Input: part model. Units: mm. Frame: model coordinates. Give positions to 0.01 mm unless a question says otherwise; leave off trailing zeros. Loops run counter-clockwise (first coordinate to the right, second up) from the corner with the lowest first, then second, coordinate; pieces in that order, holes last. Notation, with made-up numbers: (-6, 6.5) -> (5, 6.5) arc R15 cw to (5, 25.5) -> close; hole circle Ø2 at (-7, -15.5). An arc over 180 degrees is marked (long way). Answer as a JSON object with one key per item and string values. Group by question number.
```python
from build123d import *

# Parameters (mm, degrees)
SKETCH1_W           = 38.1
SKETCH1_H           = 406.4
BOSS_EXTRUDE1_DEPTH = 6.35
SKETCH2_W           = 6.35
SKETCH2_H           = 12.7
CUT_EXTRUDE1_DEPTH  = 7.35
LPATTERN1_COUNT     = 16
LPATTERN1_PITCH     = 25.4


with BuildPart() as part:
    # Sketch1 → Boss-Extrude1 (new body)
    with BuildSketch(Plane(origin=(0, 0, 0), x_dir=(0, 0, -1), z_dir=(1, 0, 0))):
        with Locations((19.05, 203.2)):
            Rectangle(SKETCH1_W, SKETCH1_H)
    extrude(amount=BOSS_EXTRUDE1_DEPTH)

    # Sketch2 → Cut-Extrude1 (cut, through all)
    with BuildSketch(Plane(origin=(6.35, 0, 0), x_dir=(0, 0, -1), z_dir=(1, 0, 0))):
        with Locations((3.175, 6.35)):
            Rectangle(SKETCH2_W, SKETCH2_H)
        with Locations((34.925, 6.35)):
            Rectangle(SKETCH2_W, SKETCH2_H)
    cut_extrude1 = extrude(amount=-CUT_EXTRUDE1_DEPTH, mode=Mode.SUBTRACT)

    # LPattern1: Cut-Extrude1 ×16
    with Locations(*[(0, i * LPATTERN1_PITCH, 0) for i in range(1, LPATTERN1_COUNT)]):
        add(cut_extrude1, mode=Mode.SUBTRACT)


solid = part.part
```
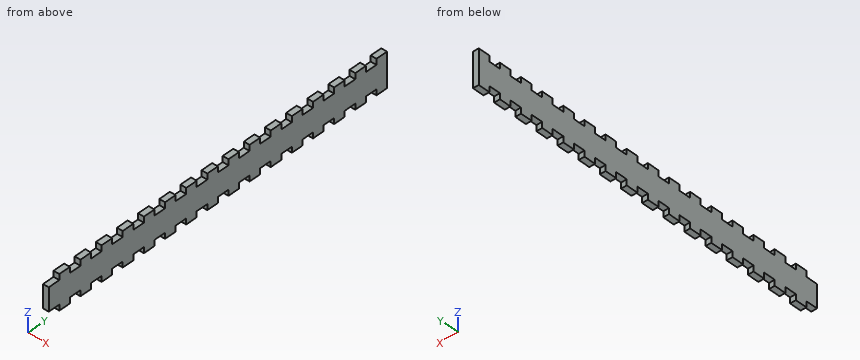
Q1. Pin query (flat end, axial travel): pin 1 Ø1 at (x, y) = (2, 207) entering from +Z; pin 2 Ø2 at (y, z) = (345.5, -17.5) entering from -X; pin 3 Ø3 at (x, z) = (4.5, -3) entering from -Y. Return the tip coordinate at first contact, or that it passes through.
Q2. Ray query, probe 1 along Z at (x, y) = (3.25, 154). Return the intervals inside material, ascending.
Q3. Section A-A on y = 261.5. Return the cut outline in (x, z), then the cut area to 3 significant figures.
Numbers:
{
 "1": {"pin 1": "stops at z = -6.35", "pin 2": "stops at x = 0", "pin 3": "stops at y = 12.7"},
 "2": {"probe 1": "z = -31.75 to -6.35"},
 "3": {"outline": "(0, -31.75) -> (6.35, -31.75) -> (6.35, -6.35) -> (0, -6.35) -> close", "area": "161 mm²"}
}
